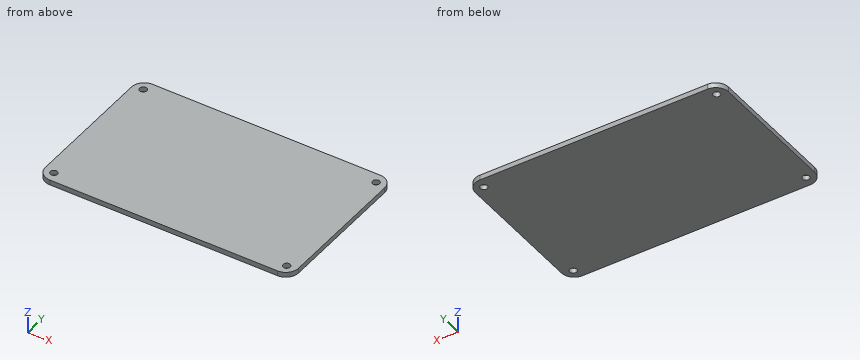
from build123d import *

# Parameters (mm, degrees)
SKETCH_1_W      = 100
SKETCH_1_H      = 62
SKETCH_1_R      = 1.4
EXTRUDE_1_DEPTH = 2
FILLET_1_R      = 5


with BuildPart() as part:
    # 草图1 → 凸台-拉伸1 (new body)
    with BuildSketch(Plane.XY):
        with Locations((50, 31)):
            Rectangle(SKETCH_1_W, SKETCH_1_H)
        with Locations((4, 58)):
            Circle(SKETCH_1_R, mode=Mode.SUBTRACT)
        with Locations(Location((4, 4, 0), (0, 0, 180))):
            Circle(SKETCH_1_R, mode=Mode.SUBTRACT)
        with Locations((96, 4)):
            Circle(SKETCH_1_R, mode=Mode.SUBTRACT)
        with Locations(Location((96, 58, 0), (0, 0, 180))):
            Circle(SKETCH_1_R, mode=Mode.SUBTRACT)
    extrude(amount=EXTRUDE_1_DEPTH)

    # 圆角1
    fillet_1_edges = [part.edges().sort_by_distance(p)[0] for p in [
        (0, 62, 1),
        (100, 62, 1),
        (100, 0, 1),
        (0, 0, 1),
    ]]
    fillet(fillet_1_edges, radius=FILLET_1_R)


solid = part.part
Could you check a few things on this model? Use its own coordinates, in mm. Give positions to 0.01 mm unless a question says otherwise; leave off trailing zeros. Order: outer loops, then holes, each group sorted by start corner. A loop starts at its lowest first (then second) coordinate and runs counter-clockwise, first axis right, second up.
Item 1: If we section it at A-A, the plane x = 4: Write out the boundary of the cut face in (y, z), plus the area to 3 significant figures.
Item 2: I need wall thicknesses on line 1 (Y direction, x = 4, z = 1.3). Which ranges of the line are inside material? Lowest first, please.
Item 3: If we section it at B-B, the plane y = 4: Write out the boundary of the cut face in (x, z).
Item 4: I'm going to push a flat-ended pin straight in: pin 1 (1.7 mm diameter, centred on x = 96, y = 4, fed in from +Z). Where does the tip first touch, or does it pass through?
Values:
1. outline: (0.1, 0) - (2.6, 0) - (2.6, 2) - (0.1, 2) - close; (5.4, 0) - (56.6, 0) - (56.6, 2) - (5.4, 2) - close; (59.4, 0) - (61.9, 0) - (61.9, 2) - (59.4, 2) - close
1. area: 112 mm2
2. line 1: y = 0.1 to 2.6, 5.4 to 56.6, 59.4 to 61.9
3. outline: (0.1, 0) - (2.6, 0) - (2.6, 2) - (0.1, 2) - close; (5.4, 0) - (94.6, 0) - (94.6, 2) - (5.4, 2) - close; (97.4, 0) - (99.9, 0) - (99.9, 2) - (97.4, 2) - close
4. pin 1: passes through
